Could you check a few things on this drawing? It's one solid part, dimensions in mm from its lowest x, y, z. A direction names the side the tool comes from. Give positions to 0.01 mm unless a question says otherwise; leave off trailing zeros. Loops run counter-clockwise (first coordinate to the right, second up) from the corner with the lowest first, then second, coordinate; pieces in that order, holes last. Notation, with made-up numbers: M 82,82.5 L 103,82.5 A23 ccw 103,115.5 Z; hole C 63.5,-8 d10. An arc over 180 degrees is marked long. Return JSON: item names as keys, results as strings. Group by question number.
1. Please list where these lines run through material, in increasing order: line 1 (Z direction, x = 20, y = 62); line 2 (X direction, y = 6.5, z = 211); line 3 (Y direction, x = 46, z = 77).
2. If we section it at A-A (z = 20): Write out the boundary of the cut face in (x, y).
3. If we section it at D-D (z = 415): Write out the boundary of the cut face in (x, y).
4. For the marked faces 1, 2 and 3, which set-ups out of +Z, -Z, +X, -X, +Y, -Y let a thin tool reach every point of the face, with its end or its side?
5. If we section it at B-B (x = 95): Write out the boundary of the cut face in (y, z), plus the area to 3 significant figures.
6. For pin 1 (12 mm diameter, centred on y = 20, z = 400.5, fed in from +X); pin 2 (5 mm diameter, centred on x = 67, y = 67, fed in from +Z); pin 3 (11 mm diameter, centred on x = 59, z = 261.5, fed in from +Y), each with a flat end and sliding along its axis, tell me the tip position at first contact or that it passes through.
7. If we section it at C-C (y = 21.5): Write out the boundary of the cut face in (x, z), plus the area to 3 significant figures.
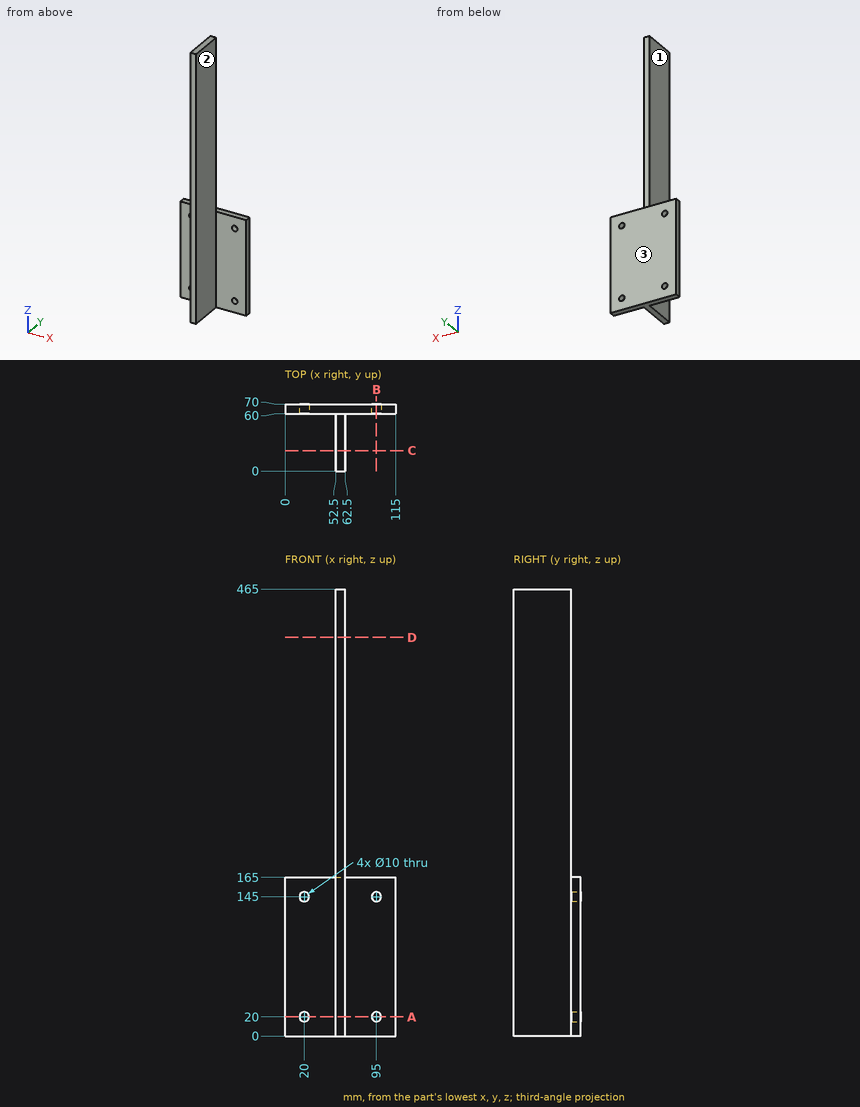
Answer:
{
 "1": {"line 1": "z = 0 to 15, 25 to 140, 150 to 165", "line 2": "x = 52.5 to 62.5", "line 3": "y = 60 to 70"},
 "2": {"outline": "M 0,60 L 15,60 L 15,70 L 0,70 Z; M 25,60 L 52.5,60 L 52.5,0 L 62.5,0 L 62.5,60 L 90,60 L 90,70 L 25,70 Z; M 100,60 L 115,60 L 115,70 L 100,70 Z"},
 "3": {"outline": "M 52.5,0 L 62.5,0 L 62.5,60 L 52.5,60 Z"},
 "4": {"face 1": "+Z, -Z, -X, -Y", "face 2": "+Z, -Z, +X, -Y", "face 3": "+Z, -Z, +X, -X, +Y"},
 "5": {"outline": "M 60,0 L 70,0 L 70,15 L 60,15 Z; M 60,25 L 70,25 L 70,140 L 60,140 Z; M 60,150 L 70,150 L 70,165 L 60,165 Z", "area": "1,450 mm²"},
 "6": {"pin 1": "stops at x = 62.5", "pin 2": "stops at z = 165", "pin 3": "stops at y = 60"},
 "7": {"outline": "M 52.5,0 L 62.5,0 L 62.5,465 L 52.5,465 Z", "area": "4,650 mm²"}
}
